Geometry check sheet. Reference: the model listing, model coordinates, mm. A direction names the side the tool comes from. Give positions to 0.01 mm unless a question says otherwise; leave off trailing zeros. Write each loop counter-clockwise with the first axis right and the second up, starting at its lowest first coordinate (ties: lowest second). Pieces come first, ordered by that corner, then holes. Notation, with made-up numbers: M 79,2 L 83,2 A14 ccw 83,6 Z; hole C 30,36.25 d4. An arc over 180 degrees is marked long. One line per item, written item: value. Start each with the question number.
1. Cross-section at A-A on x = 16.5. Record the cut outline in (y, z).
2. Cross-section at D-D on y = -9.5. Record the cut outline in (x, z), then the cut area to 3 significant figures.
3. Release check for a two-part mould opening along X. For faces 1 (the face through (35.694, -9.521, -4.686)), 2 (the face through (-13, -14, -32)), 3 (the face through (-41, -5.5, -3.3)) record: pulls with the +X half, pulls with the -X half, needs draft (parallel to the pull), parting line crosses it, or undercut.
4. Cross-section at B-B on z = 10.5. Record the cut outline in (x, y) (3 decimals).
5. Gauge pin test, flat ends, axial feed: pin 1 (10 mm diameter, centred on x = 2.5, z = -19, fed in from +Y); pin 2 (2 mm diameter, centred on y = -1.5, z = -10.5, fed in from -X); pin 3 (5 mm diameter, centred on x = -0.5, z = 42, fed in from +Y); pin 4 (5 mm diameter, centred on x = 40.9, z = 0, fed in from -Y). Record the tip position at first contact, or that the pin passes through.
6. Cross-section at C-C on y = -2. Record the cut outline in (x, z).
7. Scan lines: line 1 (Y direction, x = 14, z = 18); line 2 (Z direction, x = 40.9, y = -3.15); line 3 (Z direction, x = -40.9, y = -6.8). Record each from-to range of solid material in increasing order.
8. Tool access check on faces 4 (the face through (-13, -11, 32)), 5 (the face through (-32, -8, 18)), 6 (the face through (-41.98, -2.71, -4.88)), 7 (the face through (-21.477, -11.451, -4.769)). Record the directions out of +Z, -Z, +X, -X, +Y, -Y that give a thin tool (end or side, any length) a straight path to the whole face; none if there is none.
from build123d import *

# Parameters (mm, degrees)
F2_R     = 5
F2_R_2   = 3
F3_DEPTH = 5.5
F4_DEPTH = 25


with BuildPart() as f1:
    # F0 (on Right) → F1 (revolve)
    with BuildSketch(Plane.YZ):
        Polygon((-8, 28.65), (0, 28.65), (0, 47.9), (-8, 47.9), (-8, 36), (-11, 36), (-11, 34), (-14, 34), (-14, 36), (-15, 36), (-15, 22), (-8, 22), align=None)
    revolve(axis=Axis((0, 0.8244532039, 0), (0, 1, 0)))

    # F2 (on Front) → F3 (cut)
    with BuildSketch(Plane.XZ):
        with Locations((0, 40.9)):
            Circle(F2_R)
        with Locations((0, 40.9)):
            Circle(F2_R_2, mode=Mode.SUBTRACT)
        with Locations((-40.9, 0)):
            Circle(F2_R)
        with Locations((-40.9, 0)):
            Circle(F2_R_2, mode=Mode.SUBTRACT)
        with Locations((40.9, 0)):
            Circle(F2_R)
        with Locations((40.9, 0)):
            Circle(F2_R_2, mode=Mode.SUBTRACT)
        with Locations((0, -40.9)):
            Circle(F2_R)
        with Locations((0, -40.9)):
            Circle(F2_R_2, mode=Mode.SUBTRACT)
    extrude(amount=F3_DEPTH, mode=Mode.SUBTRACT)

    # F4 (cut): faces of the model
    f4_faces = [f1.faces().sort_by_distance(p)[0] for p in [
        (-40.9, 0, 0),
        (0, 0, 40.9),
        (40.9, 0, 0),
        (0, 0, -40.9),
    ]]
    extrude(f4_faces, amount=-F4_DEPTH, mode=Mode.SUBTRACT)


solid = f1.part
Report:
1. outline: M -15,-32 L -14,-32 L -14,-29.73 L -11,-29.73 L -11,-32 L -8,-32 L -8,-44.97 L 0,-44.97 L 0,-23.42 L -8,-23.42 L -8,-14.55 L -15,-14.55 Z; M -15,14.55 L -8,14.55 L -8,23.42 L 0,23.42 L 0,44.97 L -8,44.97 L -8,32 L -11,32 L -11,29.73 L -14,29.73 L -14,32 L -15,32 Z
2. outline: C 0,0 d72; hole C 0,0 d44
2. area: 2,550 mm^2
3. face 1: parting line crosses it
3. face 2: needs draft
3. face 3: undercut
4. outline: M -46.735,-8 L -34.435,-8 L -34.435,-11 L -32.338,-11 L -32.338,-14 L -34.435,-14 L -34.435,-15 L -19.333,-15 L -19.333,-8 L -26.657,-8 L -26.657,0 L -46.735,0 Z; M 19.333,-15 L 34.435,-15 L 34.435,-14 L 32.338,-14 L 32.338,-11 L 34.435,-11 L 34.435,-8 L 46.735,-8 L 46.735,0 L 26.657,0 L 26.657,-8 L 19.333,-8 Z
5. pin 1: stops at y = -8
5. pin 2: stops at x = -46.95
5. pin 3: stops at y = -5.5
5. pin 4: passes through
6. outline: C 0,0 d95.8; hole C -40.9,0 d10; hole C 0,0 d57.3; hole C 0,-40.9 d10; hole C 0,40.9 d10; hole C 40.9,0 d10
7. line 1: y = -15 to -8
7. line 2: z = -24.93 to -5, 5 to 24.93
7. line 3: z = -24.93 to -3, 3 to 24.93
8. face 4: none
8. face 5: -Y
8. face 6: +Y
8. face 7: +Y, -Y
